Design review of the part shown in the three views and the two pictorial views. Dimensions are in mm from the part's minimum x, y and z. Round coordinates to 2 decimals unless told otherwise and drop trailing zeros. Order: outer loops, then holes, each group sorted by start corner. A loop starts at its lowest first (then second) coordinate and runs counter-clockwise, first axis right, second up.
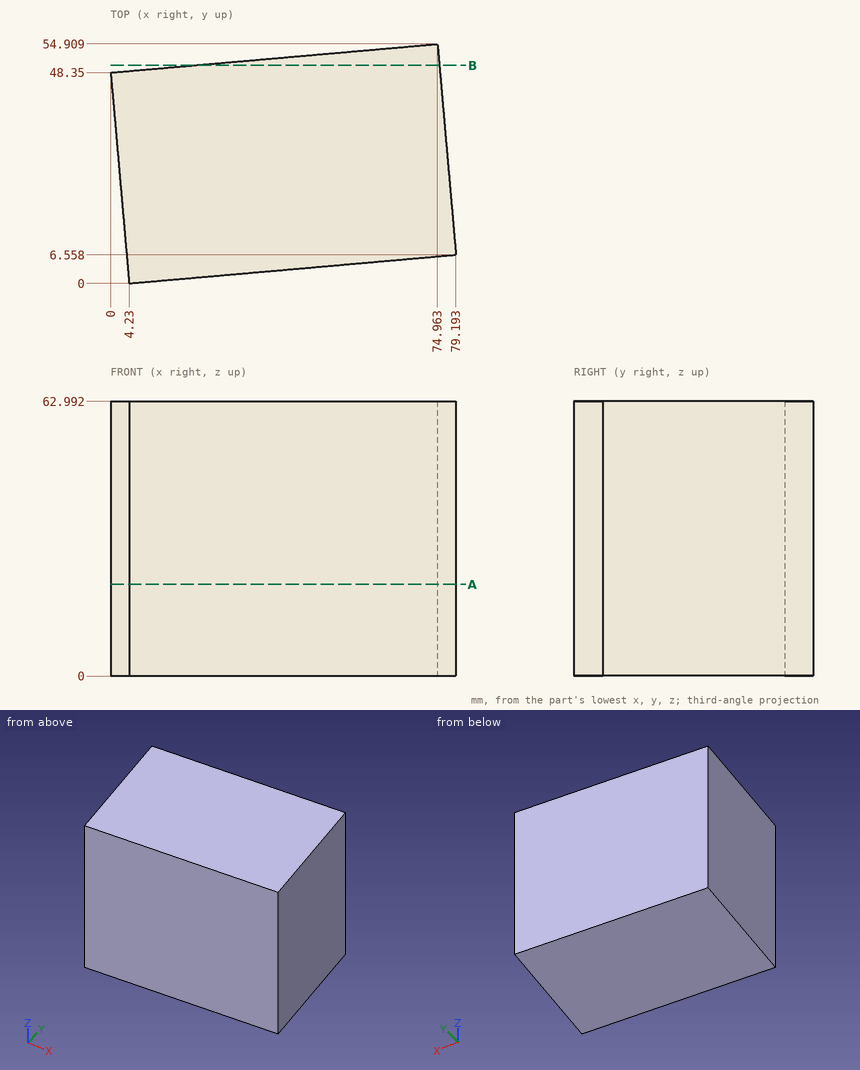
(1) Insertion check: pin 1 (12 mm diameter, centred on x = 13.5, z = 14.5, fed in from -Y); pin 2 (1.5 mm diameter, centred on y = 47, z = 18, fed in from +X); pin 3 (6 mm diameter, centred on x = 43.5, z = 11, fed in from -Y). Each pin has a flat end and moves straight along its axis. Give the tip position at first contact, or say it passes through.
Data:
pin 1: stops at y = 0.29
pin 2: stops at x = 75.72
pin 3: stops at y = 3.17
(2) Consider section A-A (z = 21). Write out the cut boundary in (x, y), and give its area (3 significant figures).
Data:
outline: (0, 48.35) - (4.23, 0) - (79.19, 6.56) - (74.96, 54.91) - close
area: 3,650 mm2
(3) Consider section B-B (y = 50). Write out the cut boundary in (x, z), and give its area (3 significant figures).
Data:
outline: (18.86, 0) - (75.39, 0) - (75.39, 62.99) - (18.86, 62.99) - close
area: 3,560 mm2
(4) To check wall thickness, follow probe 1 along Y at (x, z) = (38.5, 9.5); probe 2 along Y at (x, z) = (37.5, 8.5); probe 3 along X at (y, z) = (31, 15) (1 decimal). State the ranges of each line that lie inside material, in increasing order.
Data:
probe 1: y = 3 to 51.72
probe 2: y = 2.91 to 51.63
probe 3: x = 1.5 to 77.1
